CAD build for the part. Positions are in the model's coordinates, mm. Face numbers are marked on the shaded views. A direction names the side the tool comes from. Give positions to 0.01 mm unless a question says otherwise; leave off trailing zeros. Loops run counter-clockwise (first coordinate to the right, second up) from the corner with the lowest first, then second, coordinate; pieces in that order, holes last. Notation, with made-up numbers: M 82,69.25 L 136,69.25 A10 cw 136,83.25 Z; hole C -1,33 d9. An arc over 180 degrees is marked long. Answer as CSV lines item,"result".
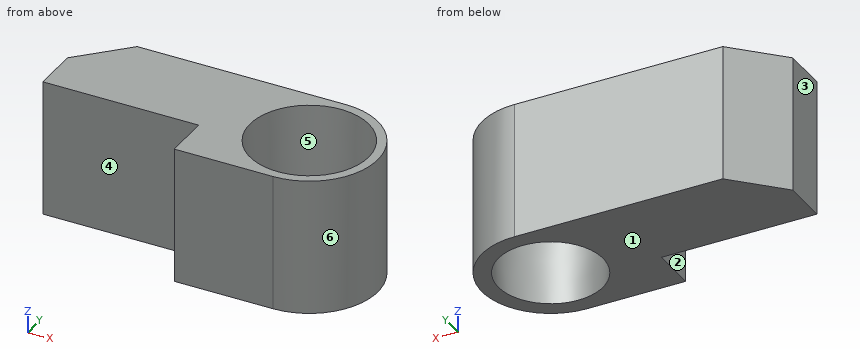
from build123d import *

# Parameters (mm, degrees)
F1_DEPTH = 15
F2_R     = 6.5
F3_DEPTH = 15
F3_TAPER = 3
F4_SIZE  = 5


with BuildPart() as f1:
    # F0 (on Top) → F1 (new body)
    with BuildSketch(Plane.XY):
        with BuildLine():
            Line((-10, -5), (7, -5))
            Line((7, -5), (7, -10))
            Line((7, -10), (10, -10))
            Line((10, -10), (17.7848991007, -10))
            ThreePointArc((17.7848991007, -10), (25.2848991007, -2.5), (17.7848991007, 5))
            Line((17.7848991007, 5), (10, 5))
            Line((10, 5), (-10, 5))
            Line((-10, 5), (-10, -5))
        make_face()
    extrude(amount=F1_DEPTH)

    # F2 (on face) → F3 (cut, through all)
    with BuildSketch(Plane.XY.offset(15)):
        with Locations((17.7848991007, -2.5)):
            Circle(F2_R)
    extrude(amount=-F3_DEPTH, taper=F3_TAPER, mode=Mode.SUBTRACT)

    # F4
    f4_edges = [f1.edges().sort_by_distance(p)[0] for p in [
        (-10, 5, 7.5),
    ]]
    chamfer(f4_edges, length=F4_SIZE)


solid = f1.part
1) Band-saw the part on A-A on z = 12.75. Give the cut face in (x, y).
Answer below:
outline,"M -10,-5 L 7,-5 L 7,-10 L 17.78,-10 A7.5 ccw 17.78,5 L -5,5 L -10,0 Z; hole C 17.78,-2.5 d12.76"
2) Which spindle directions (+Z, -Z, +X, -X, +Y, -Y) get a long thin tool onto all of the face, cutting with end or side? Do the marked faces 1 and 2. Say none if no direction does.
Answer below:
face 1,"-Z, +X, -X, +Y, -Y"
face 2,"+Z, -Z, -X, -Y"
3) Band-saw the part on B-B on x = 4. Give the cut face in (y, z), and give its area (3 significant figures).
Answer below:
outline,"M -5,0 L 5,0 L 5,15 L -5,15 Z"
area,"150 mm^2"
4) Drill centre lines: line 1 (Y direction, x = 21.5, z = 5.5); line 2 (X direction, y = -6.25, z = 14); line 3 (Y direction, x = -4.5, z = 6.25). Where is each one in solid material? Low to high. Write a range as from..to.
Answer below:
line 1,"y = -9.02..-7.21, 2.21..4.02"
line 2,"x = 7..12.54, 23.03..24.28"
line 3,"y = -5..5"
5) Mould opens along X. For the marked faces 3, 4, 5 and 6 say: +X half, -X half, draft (parallel to the pull), parting line (faces both ways), or undercut.
Answer below:
face 3,"-X half"
face 4,"draft"
face 5,"undercut"
face 6,"+X half"
6) Band-saw the part on C-C on z = 5.25. Give the cut face in (x, y), and give its area (3 significant figures).
Answer below:
outline,"M -10,-5 L 7,-5 L 7,-10 L 17.78,-10 A7.5 ccw 17.78,5 L -5,5 L -10,0 Z; hole C 17.78,-2.5 d11.98"
area,"295 mm^2"
7) Flat gauge pins, fed straight in: pin 1 (2 mm diameter, centred on y = -6.5, z = 4.5, fed in from -X); pin 2 (7.5 mm diameter, centred on x = 0.5, z = 6.5, fed in from -Y); pin 3 (6 mm diameter, centred on y = 1.5, z = 11.5, fed in from +X). Where does each tip first touch, or does it go through?
Answer below:
pin 1,"stops at x = 7"
pin 2,"stops at y = -5"
pin 3,"stops at x = 25.22"
